from build123d import *

# Parameters (mm, degrees)
CROQUIS1_R               = 1.65
CROQUIS1_R_2             = 11.4
SALIENTE_EXTRUIR1_DEPTH  = 6
SALIENTE_EXTRUIR2_DEPTH  = 6
NERVIO1_REACH            = 48.685
CROQUIS3_WALL_W          = 107.170654524
CROQUIS3_WALL_H          = 10
SALIENTE_EXTRUIR3_DEPTH  = 2
REDONDEO1_R              = 20
REDONDEO1_OF_SIMETR_A1_R = 20


with BuildPart() as part:
    # Croquis1 → Saliente-Extruir1 (new body)
    with BuildSketch(Plane.XY):
        Polygon((-21.5, -21.5), (21.5, -21.5), (21.5, 17.5), (17.5, 21.5), (-17.5, 21.5), (-21.5, 17.5), align=None)
        with Locations((-15.6, 15.6)):
            Circle(CROQUIS1_R, mode=Mode.SUBTRACT)
        with Locations((-15.6, -15.6)):
            Circle(CROQUIS1_R, mode=Mode.SUBTRACT)
        with Locations(Location((15.6, -15.6, 0), (0, 0, 180))):
            Circle(CROQUIS1_R, mode=Mode.SUBTRACT)
        with Locations(Location((15.6, 15.6, 0), (0, 0, 180))):
            Circle(CROQUIS1_R, mode=Mode.SUBTRACT)
        Circle(CROQUIS1_R_2, mode=Mode.SUBTRACT)
    extrude(amount=SALIENTE_EXTRUIR1_DEPTH)

    # Croquis2 → Saliente-Extruir2 (add)
    with BuildSketch(Plane.XZ.offset(21.5)):
        with BuildLine():
            Line((-21.5, 0), (21.5, 0))
            Line((21.5, 0), (21.5, 26))
            ThreePointArc((21.5, 26), (20.035533906, 29.535533906), (16.5, 31))
            Line((16.5, 31), (-16.5, 31))
            ThreePointArc((-16.5, 31), (-20.035533906, 29.535533906), (-21.5, 26))
            Line((-21.5, 26), (-21.5, 0))
        make_face()
    extrude(amount=SALIENTE_EXTRUIR2_DEPTH)

    # Croquis3 wall → Nervio1 (add, up to next)
    with BuildSketch(Plane(origin=(0, -16.75, 9.5), x_dir=(0, -0.805055837353, 0.59319903805), z_dir=(0, -0.59319903805, -0.805055837353)), mode=Mode.PRIVATE) as nervio1_sk1:
        Rectangle(CROQUIS3_WALL_W, CROQUIS3_WALL_H)
    nervio1_tool1 = extrude(nervio1_sk1.sketch, amount=NERVIO1_REACH, mode=Mode.PRIVATE) - part.part
    add(nervio1_tool1.solids().sort_by_distance((0, -16.75, 9.5))[0])

    # Croquis4 → Saliente-Extruir3 (add)
    with BuildSketch(Plane(origin=(21.5, 0, 0), x_dir=(0, 0, -1), z_dir=(1, 0, 0))):
        Polygon((-6, -21.5), (-6, 6.5), (-16, -21.5), align=None)
        Polygon((-26, -27.5), (0, -27.5), (0, 17.5), (-6, 17.5), (-6, -21.5), (-26, -21.5), align=None)
    saliente_extruir3 = extrude(amount=SALIENTE_EXTRUIR3_DEPTH)

    # Redondeo1
    # the kernel refuses this fillet: 20 mm, written as the material it takes off along each edge
    with BuildSketch(Plane(origin=(23.5, 17.5, -21.794494718), x_dir=(0, -1, 0), z_dir=(0, 0, 1)), Plane(origin=(23.5, 0.294494718, 26), x_dir=(0, 0, -1), z_dir=(0, -1, 0))) as redondeo1_piece_1:
        with BuildLine():
            CenterArc((8.717797887, -20), REDONDEO1_R, 90, 25.841932763)
            Line((0, -2), (-0.174355958, -1.64))
            ThreePointArc((-0.174355958, -1.64), (-0.4, -1), (-0.4, 0))
            Line((-0.4, 0), (0, 0.4))
            Line((0, 0.4), (8.717797887, 0.4))
            Line((8.717797887, 0.4), (8.717797887, 0))
        make_face()
    extrude(amount=49.588989435, mode=Mode.SUBTRACT)

    # Simetría1: Saliente-Extruir3 across plane
    add(saliente_extruir3.mirror(Plane(origin=(0, 0, 0), x_dir=(0, 0, 1), z_dir=(1, 0, 0))))

    # Redondeo1 of Simetría1
    # the kernel refuses this fillet: 20 mm, written as the material it takes off along each edge
    with BuildSketch(Plane(origin=(-23.5, 17.5, -21.794494718), x_dir=(0, -1, 0), z_dir=(0, 0, 1))) as redondeo1_of_simetr_a1_piece_1:
        with BuildLine():
            CenterArc((8.717797887, 20), REDONDEO1_OF_SIMETR_A1_R, 244.158067237, 25.841932763)
            Line((0, 2), (-0.174355958, 1.64))
            ThreePointArc((-0.174355958, 1.64), (-0.4, 1), (-0.4, 0))
            Line((-0.4, 0), (0, -0.4))
            Line((0, -0.4), (8.717797887, -0.4))
            Line((8.717797887, -0.4), (8.717797887, 0))
        make_face()
    extrude(amount=49.588989435, mode=Mode.SUBTRACT)
    with BuildSketch(Plane(origin=(-23.5, 0.294494718, 26), x_dir=(1, 0, 0), z_dir=(0, -1, 0))) as redondeo1_of_simetr_a1_piece_2:
        with BuildLine():
            CenterArc((20, -8.717797887), REDONDEO1_OF_SIMETR_A1_R, 154.158067237, 25.841932763)
            Line((0, -8.717797887), (-0.4, -8.717797887))
            Line((-0.4, -8.717797887), (-0.4, 0))
            Line((-0.4, 0), (0, 0.4))
            ThreePointArc((0, 0.4), (1, 0.4), (1.64, 0.174355958))
            Line((1.64, 0.174355958), (2, 0))
        make_face()
    extrude(amount=49.588989435, mode=Mode.SUBTRACT)


solid = part.part
Verification items for the finished model (mm, model axes). A direction names the side the tool comes from. Coordinates: 2 decimals unless noted, no trailing zeros. Order: outer loops, then holes, each group sorted by start corner. A loop starts at its lowest first (then second) coordinate and runs counter-clockwise, first axis right, second up.
Item 1: Section check D-D, the plane x = 15.6. Enter the section's corners in (y, z).
Filled in:
outline: (-27.5, 0) - (-17.25, 0) - (-17.25, 6) - (-21.5, 6) - (-21.5, 31) - (-27.5, 31) - close; (-13.95, 0) - (13.95, 0) - (13.95, 6) - (-13.95, 6) - close; (17.25, 0) - (21.5, 0) - (21.5, 6) - (17.25, 6) - close
Item 2: Access from +Z, -Z, +X, -X, +Y, -Y to the whole of each face (thin tool, end or side, straight path). Record for faces 1 (the face through (14, 16, 3)), 2 (the face through (5, -19, 9)).
Filled in:
face 1: +Z, -Z
face 2: +Z, +Y
Item 3: Section check B-B, the plane y = -4.5. Enter the section's corners in (x, z), then the cut area to 3 significant figures.
Filled in:
outline: (-23.5, 0) - (-10.47, 0) - (-10.47, 6) - (-21.5, 6) - (-21.5, 9.93) - (-23.5, 9.93) - close; (10.47, 0) - (23.5, 0) - (23.5, 9.93) - (21.5, 9.93) - (21.5, 6) - (10.47, 6) - close
area: 172 mm2
Item 4: Section check C-C, the plane z = 2. Enter the section's corners in (x, y).
Filled in:
outline: (-23.5, -27.5) - (23.5, -27.5) - (23.5, 8.78) arc R20 ccw to (21.5, 17.5) - (17.5, 21.5) - (-17.5, 21.5) - (-21.5, 17.5) arc R20 ccw to (-23.5, 8.78) - close; hole circle Ø3.3 at (-15.6, -15.6); hole circle Ø3.3 at (-15.6, 15.6); hole circle Ø22.8 at (0, 0); hole circle Ø3.3 at (15.6, -15.6); hole circle Ø3.3 at (15.6, 15.6)
Item 5: Section check A-A, the plane x = 0. Enter the section's corners in (y, z).
Filled in:
outline: (-27.5, 0) - (-11.4, 0) - (-11.4, 6) - (-12, 6) - (-21.5, 13) - (-21.5, 31) - (-27.5, 31) - close; (11.4, 0) - (21.5, 0) - (21.5, 6) - (11.4, 6) - close
Item 6: Material ranges on L1, parallel to Y at x = 15.6, z = 2.1; L2, parallel to X at y = -21, z = 9.5; L3, parallel to X at y = 15, z = 2, recorded low to high.
Filled in:
L1: y = -27.5 to -17.25, -13.95 to 13.95, 17.25 to 21.5
L2: x = -23.5 to -21.5, -5 to 5, 21.5 to 23.5
L3: x = -22.51 to -17.14, -14.06 to 14.06, 17.14 to 22.51
Item 7: Release check for a two-part mould opening along Y. For faces 3 (the face through (14.076, -14.968, 2.958)), 4 (the face through (-20, -24.46, 29.57)), 5 (the face through (20, 19, 3)) record: +Y half, -Y half, draft (parallel to the pull), parting line (faces both ways), or undercut.
Filled in:
face 3: undercut
face 4: draft
face 5: +Y half
Item 8: Depth check by flat-ended pin: pin 1 (10 mm diameter, centred on x = -2.5, y = -6.5, fed in from -Z); pin 2 (5 mm diameter, centred on x = 12.5, y = -16, fed in from +Z); pin 3 (21.5 mm diameter, centred on x = 0.5, y = -3.5, fed in from +Z); pin 4 (12.5 mm diameter, centred on x = 2, z = 24.5, fed in from +Y). Enter the tip coordinate at first touch or a pass-through.
Filled in:
pin 1: stops at z = 0
pin 2: stops at z = 6
pin 3: stops at z = 7.66
pin 4: stops at y = -21.5
